from build123d import *

# Parameters (mm, degrees)
SKETCH_1_W                       = 3
SKETCH_1_H                       = 30
SM_BASE_FLANGE_1_DEPTH           = 240
SKETCH_6_R                       = 4.25
CUT_EXTRUDE_1_DEPTH              = 242.886336944
SM_EDGE_FLANGE_1_STRIP_W         = 15
SM_EDGE_FLANGE_1_STRIP_H         = 3
SM_EDGE_FLANGE_1_STRIP_CUT_DEPTH = 240
SM_EDGE_FLANGE_1_DEPTH           = 240


# Sheet-metal steps are written as plain solids
with BuildPart() as part:
    # Sketch 1 → Базовая кромка1 (new body)
    with BuildSketch(Plane.XY):
        with Locations((1.5, -15)):
            Rectangle(SKETCH_1_W, SKETCH_1_H)
    extrude(amount=-SM_BASE_FLANGE_1_DEPTH)

    # Эскиз6 → Вырез-Вытянуть1 (cut, through all)
    with BuildSketch(Plane(origin=(3, 0, 0), x_dir=(0, 0, -1), z_dir=(1, 0, 0))):
        with Locations(Location((225, -15, 0), (0, 0, 90))):
            Circle(SKETCH_6_R)
        with Locations(Location((165, -15, 0), (0, 0, 90))):
            Circle(SKETCH_6_R)
        with Locations(Location((75, -15, 0), (0, 0, 90))):
            Circle(SKETCH_6_R)
        with Locations(Location((15, -15, 0), (0, 0, 90))):
            Circle(SKETCH_6_R)
    extrude(amount=-CUT_EXTRUDE_1_DEPTH, mode=Mode.SUBTRACT)

    # Ребро-кромка1 strip (across the edge) → Ребро-кромка1 strip cut (cut)
    with BuildSketch(Plane(origin=(0, 0, 0), x_dir=(0, -1, 0), z_dir=(0, 0, -1))):
        with Locations((-6, -1.5)):
            Rectangle(SM_EDGE_FLANGE_1_STRIP_W, SM_EDGE_FLANGE_1_STRIP_H)
    extrude(amount=SM_EDGE_FLANGE_1_STRIP_CUT_DEPTH, mode=Mode.SUBTRACT)

    # Ребро-кромка1 section (across the edge) → Ребро-кромка1 (add)
    with BuildSketch(Plane(origin=(0, 0, 0), x_dir=(0, -1, 0), z_dir=(0, 0, -1))):
        with BuildLine():
            Line((-3, 1.5), (-3, 11))
            Line((-3, 11), (0, 11))
            Line((0, 11), (0, 1.5))
            ThreePointArc((0, 1.5), (0.439339828, 0.439339828), (1.5, 0))
            Line((1.5, 0), (1.5, -3))
            ThreePointArc((1.5, -3), (-1.681980515, -1.681980515), (-3, 1.5))
        make_face()
    extrude(amount=SM_EDGE_FLANGE_1_DEPTH)


solid = part.part
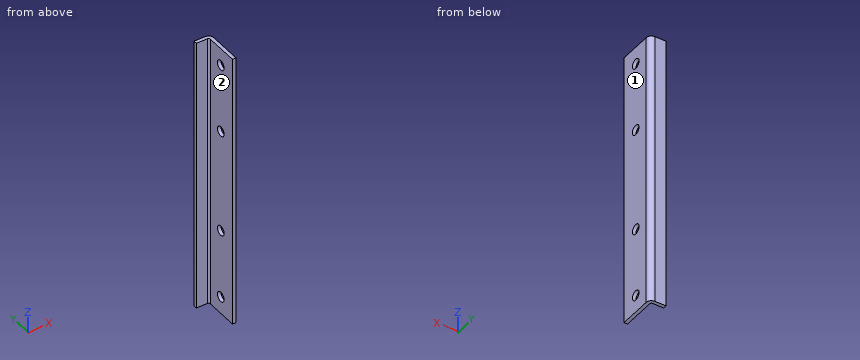
Design review of the part built by this model. Coordinates are the model's own, in mm. Face numbers are marked on the shaded views. A direction names the side the tool comes from. Coordinates: 2 decimals unless noted, no trailing zeros. Order: outer loops, then holes, each group sorted by start corner. A loop starts at its lowest first (then second) coordinate and runs counter-clockwise, first axis right, second up. Notation, with made-up numbers: (-35.5, 30) -> (15.5, 30) arc R16 cw to (15.5, 50) -> close; hole circle Ø4 at (14.25, 41). An arc over 180 degrees is marked (long way). Use one line per item in the form item = value. Start each with the question number.
(1) For probe 1 along Z at (x, y) = (2.15, -15); probe 2 along X at (y, z) = (-13.5, -194), list the stretches that pass through material, from the lowest coordinate up.
(2) Add section B-B on y = -15. State the section outline as (x, z) points.
(3) Add section A-A on z = -15. State the section outline as (x, y) points, plus the area to 3 significant figures.
(4) Add section C-C on x = -6.75. State the section outline as (y, z) points, plus the area to 3 significant figures.
(5) For the marked faces 1 and 2, list the 3-axis set-ups (+Z, -Z, +X, -X, +Y, -Y) from which the entire face can be reached by the end or side of a thin tool; tool diameter is ignored.
(6) Insertion check: pin 1 (8 mm diameter, centred on y = -5.5, z = -170, fed in from -X). The pin has a flat end and moves straight along its axis. Give the tip position at first contact, or say it passes through.
Answer block:
q1.probe_1 = -240 to -229.25, -220.75 to -169.25, -160.75 to -79.25, -70.75 to -19.25, -10.75 to 0
q1.probe_2 = 0 to 3
q2.outline = (0, -240) -> (3, -240) -> (3, -229.25) -> (0, -229.25) -> close; (0, -220.75) -> (3, -220.75) -> (3, -169.25) -> (0, -169.25) -> close; (0, -160.75) -> (3, -160.75) -> (3, -79.25) -> (0, -79.25) -> close; (0, -70.75) -> (3, -70.75) -> (3, -19.25) -> (0, -19.25) -> close; (0, -10.75) -> (3, -10.75) -> (3, 0) -> (0, 0) -> close
q3.outline = (-11, 0) -> (-1.5, 0) arc R1.5 cw to (0, -1.5) -> (0, -10.75) -> (3, -10.75) -> (3, -1.5) arc R4.5 ccw to (-1.5, 3) -> (-11, 3) -> close; (0, -30) -> (3, -30) -> (3, -19.25) -> (0, -19.25) -> close
q3.area = 103 mm²
q4.outline = (0, -240) -> (3, -240) -> (3, 0) -> (0, 0) -> close
q4.area = 720 mm²
q5.face_1 = +Z, -Z, +X, +Y, -Y
q5.face_2 = +Z, -Z, -X, -Y
q6.pin_1 = 0
